Model file for the job. Use its own axes, mm. A direction names the side the tool comes from. Coordinates: 2 decimals unless noted, no trailing zeros. Write each loop counter-clockwise with the first axis right and the second up, starting at its lowest first coordinate (ties: lowest second). Pieces come first, ordered by that corner, then holes. Notation, with made-up numbers: M 24,74.5 L 28,74.5 A18 cw 28,88.5 Z; hole C -4.75,-26 d3. An arc over 180 degrees is marked long. Answer in a Markdown table with one row per item. Add a question column.
Autodesk Inventor part; units mm, degrees
ref_plane "YZ Plane" through (0, 0, 0) normal (1, 0, 0) x (0, 1, 0)
ref_plane "XZ Plane" through (0, 0, 0) normal (0, 1, 0) x (-1, 0, 0)
ref_plane "XY Plane" through (0, 0, 0) normal (0, 0, 1) x (1, 0, 0)
sketch "Sketch1" plane through (0, 0, 0) normal (1, 0, 0) x (0, 1, 0)
  circle A0 centre (0, 0) radius 136.5
  dimension "d0" = 273
extrude "Extrusion1" add sketch "Sketch1" along normal blind 382
sketch "Sketch2" plane through (0, 0, 0) normal (0, 0, 1) x (1, 0, 0)
  line L0 (0, 136.5) -> (0, -136.5)
  line L1 (382, 136.5) -> (382, -136.5)
  line L2 (0, 0) -> (382, 0) construction
  circle A0 centre (191, 0) radius 69.85
  dimension "d3" = 139.7
extrude "Extrusion2" add sketch "Sketch2" along normal blind 191
sketch "Sketch3" plane through (0, 0, 0) normal (-1, 0, 0) x (0, 0, 1)
  circle A0 centre (0, 0) radius 136.5
  circle A1 centre (0, 0) radius 126.5
  dimension "d6" = 253
extrude "Extrusion3" cut sketch "Sketch3" against normal through all contours A1
sketch "Sketch4" plane through (191, 0, 191) normal (0, 0, 1) x (1, 0, 0)
  circle A0 centre (0, 0) radius 69.85
  circle A1 centre (0, 0) radius 63.55
  dimension "d9" = 127.1
extrude "Extrusion4" cut sketch "Sketch4" against normal up to next contours A1
equation "\"d0\" = D"
equation "\"d1\" = 2 * F1"
equation "\"d3\" = D1"
equation "\"d4\" = F1"
equation "\"d6\" = D - 2 * T"
equation "\"d7\" = F1"
equation "\"d9\" = D1 - 2 * T1"
equation "\"d10\" = F1"
equation "\"D\" = 273"
equation "\"F1\" = 191"
equation "\"D1\" = 139.7"
equation "\"T1\" = 6.3"
equation "\"Size_Designation\" = 1.2345"
properties part number "ISO 5251 Переходный тройник DN250 x DN125 10" material "Нержавеющая сталь"
1) Drill centre lines: probe 1 along Y at (x, z) = (191, 173.5); probe 2 along X at (y, z) = (0, 149); probe 3 along Z at (x, y) = (23.5, -4). Where is each one in solid material? Low to high.
2) Flat gauge pins, fed straight in: pin 1 Ø5 at (x, z) = (129.5, 81) entering from -Y; pin 2 Ø8 at (x, z) = (144, -103) entering from +Y; pin 3 Ø1 at (x, y) = (151.5, 102) entering from -Z; pin 4 Ø2 at (x, y) = (165, 57.5) entering from +Z. Where does each tip first touch, or does it go through?
3) Which spindle directions (+Z, -Z, +X, -X, +Y, -Y) get a long thin tool onto all of the face, cutting with end or side? Do faces 4 (the face through (0, 121, -40)), 5 (the face through (140.57, -38.67, 150.76)). Say none if no direction does.
4) Slice it at D-D (y = 114). Give the cut face in (x, z), then the cut area to 3 significant figures.
5) Slice it at A-A (y = 0). Give the cut face in (x, z).
6) Two-plate mould, pull along Y, no slides. Class faces 1 (the face through (206, -62, 191)), 2 (the face through (139.52, -47.21, 161.81)), 3 (the face through (188.326, 5.562, -126.378)): released by +Y, released by -Y, zero draft, split by the parting line, or undercut.
7) Slice it at C-C (x = 191). Give the cut face in (y, z).
8) Slice it at B-B (z = 0). Give the cut face in (x, y), then the cut area to 3 significant figures.
Ans:
| question | item | result |
|---|---|---|
| 1 | probe 1 | y = -69.85 to -63.55, 63.55 to 69.85 |
| 1 | probe 2 | x = 121.15 to 127.45, 254.55 to 260.85 |
| 1 | probe 3 | z = -136.44 to -126.44, 126.44 to 136.44 |
| 2 | pin 1 | stops at y = -111.67 |
| 2 | pin 2 | stops at y = 93.97 |
| 2 | pin 3 | stops at z = -91.27 |
| 2 | pin 4 | stops at z = 191 |
| 3 | face 4 | +Z, -Z, -X, +Y, -Y |
| 3 | face 5 | +Z |
| 4 | outline | M 0,-75.07 L 382,-75.07 L 382,-54.83 L 0,-54.83 Z; M 0,54.83 L 382,54.83 L 382,75.07 L 0,75.07 Z |
| 4 | area | 15,500 mm2 |
| 5 | outline | M 0,-136.5 L 382,-136.5 L 382,-126.5 L 0,-126.5 Z; M 0,126.5 L 127.45,126.5 L 127.45,191 L 121.15,191 L 121.15,136.5 L 0,136.5 Z; M 254.55,126.5 L 382,126.5 L 382,136.5 L 260.85,136.5 L 260.85,191 L 254.55,191 Z |
| 6 | face 1 | zero draft |
| 6 | face 2 | split by the parting line |
| 6 | face 3 | undercut |
| 7 | outline | M -69.85,117.27 A136.5 ccw long 69.85,117.27 L 69.85,191 L 63.55,191 L 63.55,109.38 A126.5 cw long -63.55,109.38 L -63.55,191 L -69.85,191 Z |
| 8 | outline | M 0,-136.5 L 382,-136.5 L 382,-126.5 L 0,-126.5 Z; M 0,126.5 L 382,126.5 L 382,136.5 L 0,136.5 Z |
| 8 | area | 7,640 mm2 |
